from build123d import *

# Parameters (mm, degrees)
SKETCH1_R                = 5
BOSS_EXTRUDE1_DEPTH      = 22
BOSS_EXTRUDE2_DEPTH      = 5
BOSS_EXTRUDE2_DEPTH_BACK = 8
SKETCH2_W                = 80
SKETCH2_H                = 15
SKETCH2_W_2              = 79
SKETCH2_H_2              = 14


with BuildPart() as part:
    # Sketch1 → Boss-Extrude1 (new body)
    with BuildSketch(Plane(origin=(0, 0, 0), x_dir=(0, 0, -1), z_dir=(1, 0, 0))):
        Circle(SKETCH1_R)
    extrude(amount=BOSS_EXTRUDE1_DEPTH)

    # Sketch2 → Boss-Extrude2 (add, two sides: drawn at the far end of the back side and taken through both)
    with BuildSketch(Plane(origin=(0, 0, 0), x_dir=(1, 0, 0), z_dir=(0, 1, 0)).offset(-BOSS_EXTRUDE2_DEPTH_BACK)):
        with Locations((61.5, 0)):
            Rectangle(SKETCH2_W, SKETCH2_H)
        with Locations((61.5, 0)):
            Rectangle(SKETCH2_W_2, SKETCH2_H_2, mode=Mode.SUBTRACT)
    extrude(amount=BOSS_EXTRUDE2_DEPTH + BOSS_EXTRUDE2_DEPTH_BACK)


solid = part.part
Can you work these out from the model? Positions are in its coordinate system, mm. A direction names the side the tool comes from. Give positions to 0.01 mm unless a question says otherwise; leave off trailing zeros. Write each loop counter-clockwise with the first axis right and the second up, starting at its lowest first coordinate (ties: lowest second). Pieces come first, ordered by that corner, then holes. Notation, with made-up numbers: (88.5, -10.5) -> (105.5, -10.5) arc R16 ccw to (105.5, 5.5) -> close; hole circle Ø1 at (85, -13.5). An arc over 180 degrees is marked (long way). Answer as a JSON object with one key per item and string values. Group by question number.
Item 1: Suppose I cut it at B-B (x = 49). Please give me the cut outline in (y, z).
Item 2: Please list where these lines run through material, in increasing order: line 1 (X direction, y = -7.25, z = -6.5); line 2 (Z direction, x = 69.5, y = 3); line 3 (X direction, y = -1.5, z = -3.25). Write a range as [from, to].
Item 3: Suppose I cut it at A-A (z = 6). Please give me the cut outline in (x, y).
Item 4: Suppose I cut it at D-D (y = -4). Please give me the cut outline in (x, z).
Item 5: Suppose I cut it at C-C (y = 0). Please give me the cut outline in (x, z).
Item 6: For faces 4 (the face through (61.3, 5, -7.3)), 5 (the face through (10.6, -4.88, 1.08)), 6 (the face through (61, -2, -7)), which set-ups out of +Z, -Z, +X, -X, +Y, -Y let a thin tool reach every point of the face, with its end or its side?
Item 7: I'm going to push flat-ended pins straight in: P1, Ø1.5, axis at x = 63, z = -4.5, coming from the -Y side; P2, Ø1.5, axis at x = 19.5, z = 2, coming from the -Y side; P3, Ø3, axis at x = 17, z = -0.5, coming from the -Y side. Where does each tip first touch, or does it pass through?
Item 8: We'd pull the mould along X, two halves only. Please class faces 1 (the face through (61, -2, 7.5)), 2 (the face through (22, -1, 0)), 3 (the face through (0, 0, 0)): +X half, -X half, draft (parallel to the pull), parting line (faces both ways), or undercut.
Findings:
{
 "1": {"outline": "(-8, -7.5) -> (5, -7.5) -> (5, -7) -> (-8, -7) -> close; (-8, 7) -> (5, 7) -> (5, 7.5) -> (-8, 7.5) -> close"},
 "2": {"line 1": "x = [21.5, 22], [101, 101.5]", "line 2": "z = [-7.5, -7], [7, 7.5]", "line 3": "x = [0, 22], [101, 101.5]"},
 "3": {"outline": "(21.5, -8) -> (22, -8) -> (22, 5) -> (21.5, 5) -> close; (101, -8) -> (101.5, -8) -> (101.5, 5) -> (101, 5) -> close"},
 "4": {"outline": "(0, -3) -> (21.5, -3) -> (21.5, -7.5) -> (101.5, -7.5) -> (101.5, 7.5) -> (21.5, 7.5) -> (21.5, 3) -> (0, 3) -> close; hole (22, -7) -> (101, -7) -> (101, 7) -> (22, 7) -> close"},
 "5": {"outline": "(0, -5) -> (21.5, -5) -> (21.5, -7.5) -> (101.5, -7.5) -> (101.5, 7.5) -> (21.5, 7.5) -> (21.5, 5) -> (0, 5) -> close; hole (22, -7) -> (101, -7) -> (101, 7) -> (22, 7) -> close"},
 "6": {"face 4": "+Z, -Z, +X, -X, +Y", "face 5": "-X", "face 6": "+Y, -Y"},
 "7": {"P1": "passes through", "P2": "stops at y = -4.84", "P3": "stops at y = -5"},
 "8": {"face 1": "draft", "face 2": "undercut", "face 3": "-X half"}
}
